from build123d import *

# Parameters (mm, degrees)
SKETCH033_W             = 75
SKETCH033_H             = 75
PAD011_DEPTH            = 18
SKETCH034_R             = 30
SKETCH034_R_2           = 2.5
POCKET022_DEPTH         = 18
SKETCH035_R             = 34
POCKET023_DEPTH         = 4
BODY012_PLACEMENT_ANGLE = 90


with BuildPart() as part:
    # Sketch033 → Pad011 (new body)
    with BuildSketch(Plane.XY):
        Rectangle(SKETCH033_W, SKETCH033_H)
    extrude(amount=PAD011_DEPTH)

    # Sketch034 → Pocket022 (cut)
    with BuildSketch(Plane.XY.offset(18)):
        Circle(SKETCH034_R)
        with Locations((-27.5, 27.5)):
            Circle(SKETCH034_R_2)
        with Locations((27.5, 27.5)):
            Circle(SKETCH034_R_2)
        with Locations((27.5, -27.5)):
            Circle(SKETCH034_R_2)
        with Locations((-27.5, -27.5)):
            Circle(SKETCH034_R_2)
    extrude(amount=-POCKET022_DEPTH, mode=Mode.SUBTRACT)

    # Sketch035 → Pocket023 (cut)
    with BuildSketch(Plane.XY.offset(18)):
        Circle(SKETCH035_R)
    extrude(amount=-POCKET023_DEPTH, mode=Mode.SUBTRACT)


with BuildPart() as part_1:
    # Body012 placement: moved
    add(part.part.moved(Location((-149, 252, 37.5))).rotate(Axis((-149, 252, 37.5), (0, 1, 0)), BODY012_PLACEMENT_ANGLE))


solid = part_1.part
Geometry: final body of the model. Coordinates: model frame, mm. A direction names the side the tool comes from. Round coordinates to 2 decimals unless told otherwise and drop trailing zeros. Loops run counter-clockwise (first coordinate to the right, second up) from the corner with the lowest first, then second, coordinate; pieces in that order, holes last.
Q1. Access query for faces 1 (the flat face through (-140, 251, 75)), 2 (the flat face through (-135, 221.9, 35.1)). Directions: +Z, -Z, +X, -X, +Y, -Y. A direction counts if a zero-diameter tool reaches every point of the face in a straight line with its end or side. Return the directions, or none.
Q2. Pull-direction query (Z, two-part tool) for faces 3 (the flat face through (-140, 251, 0)), 4 (the flat face through (-149, 278, 55)), 5 (the cylindrical face through (-141.902, 281.745, 41.405)); classes: released by +Z, released by -Z, zero draft, split by the parting line, or undercut.
Q3. Material intervals for L1, parallel to Z at x = -136, y = 226; L2, parallel to Y at x = -133.4, z = 37.5; L3, parallel to Y at x = -136.75, z = 65, sorted ascending.
Q4. Section B-B on y = 252. Return loops of the section in (x, z).
Q5. Section C-C on x = -146.75. Return loops of the section in (y, z).
Q6. Section D-D on z = 65. Return loops of the section in (x, y), plus the area to 3 significant figures.
Q7. Pin query (flat end, axial travel): P1, Ø4.5, axis at y = 224.5, z = 65, coming from the -X side. Return the tip coordinate at first contact, or that it passes through.
Q8. Section A-A on z = 37.5. Return loops of the section in (x, y).
Evaluation:
1. face 1: +Z, +X, -X, +Y, -Y
1. face 2: +X
2. face 3: released by -Z
2. face 4: zero draft
2. face 5: undercut
3. L1: z = 0 to 8, 12 to 22.53, 52.47 to 63, 67 to 75
3. L2: y = 214.5 to 218, 286 to 289.5
3. L3: y = 214.5 to 222, 227 to 240.01, 263.99 to 277, 282 to 289.5
4. outline: (-149, 0) - (-131, 0) - (-131, 3.5) - (-135, 3.5) - (-135, 7.5) - (-149, 7.5) - close; (-149, 67.5) - (-135, 67.5) - (-135, 71.5) - (-131, 71.5) - (-131, 75) - (-149, 75) - close
5. outline: (214.5, 0) - (289.5, 0) - (289.5, 75) - (214.5, 75) - close; hole circle Ø5 at (224.5, 10); hole circle Ø60 at (252, 37.5); hole circle Ø5 at (224.5, 65); hole circle Ø5 at (279.5, 10); hole circle Ø5 at (279.5, 65)
6. outline: (-149, 214.5) - (-131, 214.5) - (-131, 222) - (-149, 222) - close; (-149, 227) - (-131, 227) - (-131, 232.01) - (-135, 232.01) - (-135, 240.01) - (-149, 240.01) - close; (-149, 263.99) - (-135, 263.99) - (-135, 271.99) - (-131, 271.99) - (-131, 277) - (-149, 277) - close; (-149, 282) - (-131, 282) - (-131, 289.5) - (-149, 289.5) - close
6. area: 674 mm2
7. P1: passes through
8. outline: (-149, 214.5) - (-131, 214.5) - (-131, 218) - (-135, 218) - (-135, 222) - (-149, 222) - close; (-149, 282) - (-135, 282) - (-135, 286) - (-131, 286) - (-131, 289.5) - (-149, 289.5) - close
